Check sheet for the modelled part. Datum: model origin and axes. Units: mm. Give positions to 0.01 mm unless a question says otherwise; leave off trailing zeros. Loops run counter-clockwise (first coordinate to the right, second up) from the corner with the lowest first, then second, coordinate; pieces in that order, holes last. Notation, with made-up numbers: M 51.25,62 L 87.25,62 A19 ccw 87.25,82 Z; hole C 54,-14 d9. An arc over 180 degrees is marked long. Use one line per item in the form item = value.
from build123d import *

# Parameters (mm, degrees)
SKETCH1_R           = 75
BOSS_EXTRUDE1_DEPTH = 3.175
CUT_EXTRUDE1_DEPTH  = 3.175
SKETCH3_R           = 1.5875
CUT_EXTRUDE2_DEPTH  = 3.175
SKETCH4_R           = 27.051
CUT_EXTRUDE3_DEPTH  = 3.175
CUT_EXTRUDE4_DEPTH  = 3.175


with BuildPart() as part:
    # Sketch1 → Boss-Extrude1 (new body)
    with BuildSketch(Plane(origin=(0, 0, 0), x_dir=(1, 0, 0), z_dir=(0, 1, 0))):
        Circle(SKETCH1_R)
    extrude(amount=BOSS_EXTRUDE1_DEPTH)

    # Sketch2 → Cut-Extrude1 (cut)
    with BuildSketch(Plane(origin=(0, 3.175, 0), x_dir=(1, 0, 0), z_dir=(0, 1, 0))):
        with BuildLine():
            Line((-56.262005909, -49.594220339), (56.262005909, -49.594220339))
            ThreePointArc((56.262005909, -49.594220339), (0, -75), (-56.262005909, -49.594220339))
        make_face()
        with BuildLine():
            Line((-56.262005909, 49.594220339), (56.262005909, 49.594220339))
            ThreePointArc((56.262005909, 49.594220339), (0, 75), (-56.262005909, 49.594220339))
        make_face()
    extrude(amount=-CUT_EXTRUDE1_DEPTH, mode=Mode.SUBTRACT)

    # Sketch3 → Cut-Extrude2 (cut)
    with BuildSketch(Plane(origin=(0, 3.175, 0), x_dir=(1, 0, 0), z_dir=(0, 1, 0))):
        with Locations((-52.180304588, 44.729838125)):
            Circle(SKETCH3_R)
        with Locations((-19.05, 44.729838125)):
            Circle(SKETCH3_R)
        with Locations((19.05, 44.729838125)):
            Circle(SKETCH3_R)
        with Locations((52.180304588, 44.729838125)):
            Circle(SKETCH3_R)
        with Locations((52.180304588, -44.729838125)):
            Circle(SKETCH3_R)
        with Locations((19.05, -44.729838125)):
            Circle(SKETCH3_R)
        with Locations((-19.05, -44.729838125)):
            Circle(SKETCH3_R)
        with Locations((-52.180304588, -44.729838125)):
            Circle(SKETCH3_R)
    extrude(amount=-CUT_EXTRUDE2_DEPTH, mode=Mode.SUBTRACT)

    # Sketch4 → Cut-Extrude3 (cut)
    with BuildSketch(Plane(origin=(0, 3.175, 0), x_dir=(1, 0, 0), z_dir=(0, 1, 0))):
        with BuildLine():
            Line((-47.315937317, 44.741895283), (-23.177806764, 24.050282215))
            ThreePointArc((-23.177806764, 24.050282215), (-19.742091457, 26.942097653), (-15.949506316, 29.346891646))
            Line((-15.949506316, 29.346891646), (-20.527078848, 40.095137229))
            ThreePointArc((-20.527078848, 40.095137229), (-22.980849122, 41.864416778), (-23.914367271, 44.741895283))
            Line((-23.914367271, 44.741895283), (-47.315937317, 44.741895283))
        make_face()
        with BuildLine():
            ThreePointArc((10.107278818, 31.835039122), (0, 33.401), (-10.107278818, 31.835039122))
            Line((-10.107278818, 31.835039122), (-14.68485135, 42.583284705))
            ThreePointArc((-14.68485135, 42.583284705), (-14.312069768, 43.627916425), (-14.185617786, 44.729838125))
            Line((-14.185617786, 44.729838125), (14.185617786, 44.729838125))
            ThreePointArc((14.185617786, 44.729838125), (14.312069768, 43.627916425), (14.68485135, 42.583284705))
            Line((14.68485135, 42.583284705), (10.107278818, 31.835039122))
        make_face()
        with BuildLine():
            ThreePointArc((15.949506316, 29.346891646), (19.742091457, 26.942097653), (23.177806764, 24.050282215))
            Line((23.177806764, 24.050282215), (47.315937317, 44.741895283))
            Line((47.315937317, 44.741895283), (23.914382214, 44.729838125))
            ThreePointArc((23.914382214, 44.729838125), (22.977294896, 41.859547352), (20.527078848, 40.095137229))
            Line((20.527078848, 40.095137229), (15.949506316, 29.346891646))
        make_face()
        Circle(SKETCH4_R)
        with BuildLine():
            Line((-23.177806764, -24.050282215), (-47.315937317, -44.741895283))
            Line((-47.315937317, -44.741895283), (-23.914382214, -44.729838125))
            ThreePointArc((-23.914382214, -44.729838125), (-22.977294896, -41.859547352), (-20.527078848, -40.095137229))
            Line((-20.527078848, -40.095137229), (-15.949506316, -29.346891646))
            ThreePointArc((-15.949506316, -29.346891646), (-19.742091457, -26.942097653), (-23.177806764, -24.050282215))
        make_face()
        with BuildLine():
            ThreePointArc((-10.107278818, -31.835039122), (0, -33.401), (10.107278818, -31.835039122))
            Line((10.107278818, -31.835039122), (14.68485135, -42.583284705))
            ThreePointArc((14.68485135, -42.583284705), (14.312069768, -43.627916425), (14.185617786, -44.729838125))
            Line((14.185617786, -44.729838125), (-14.185617786, -44.729838125))
            ThreePointArc((-14.185617786, -44.729838125), (-14.312069768, -43.627916425), (-14.68485135, -42.583284705))
            Line((-14.68485135, -42.583284705), (-10.107278818, -31.835039122))
        make_face()
        with BuildLine():
            ThreePointArc((23.177806764, -24.050282215), (19.742091457, -26.942097653), (15.949506316, -29.346891646))
            Line((15.949506316, -29.346891646), (20.527078848, -40.095137229))
            ThreePointArc((20.527078848, -40.095137229), (22.977294896, -41.859547352), (23.914382214, -44.729838125))
            Line((23.914382214, -44.729838125), (47.315937317, -44.741895283))
            Line((47.315937317, -44.741895283), (23.177806764, -24.050282215))
        make_face()
    extrude(amount=-CUT_EXTRUDE3_DEPTH, mode=Mode.SUBTRACT)

    # Sketch5 → Cut-Extrude4 (cut)
    with BuildSketch(Plane(origin=(0, 3.175, 0), x_dir=(1, 0, 0), z_dir=(0, 1, 0))):
        with BuildLine():
            Line((58.957481542, 46.357473725), (27.31053772, 19.229179141))
            ThreePointArc((27.31053772, 19.229179141), (33.401, 0), (27.31053772, -19.229179141))
            Line((27.31053772, -19.229179141), (58.957481542, -46.357473725))
            ThreePointArc((58.957481542, -46.357473725), (75, 0), (58.957481542, 46.357473725))
        make_face()
        with BuildLine():
            Line((-54.190960711, 42.271531589), (-27.31053772, 19.229179141))
            ThreePointArc((-27.31053772, 19.229179141), (-33.401, 0), (-27.31053772, -19.229179141))
            Line((-27.31053772, -19.229179141), (-54.190960711, -42.271531589))
            ThreePointArc((-54.190960711, -42.271531589), (-68.728033622, 0), (-54.190960711, 42.271531589))
        make_face()
    extrude(amount=-CUT_EXTRUDE4_DEPTH, mode=Mode.SUBTRACT)


solid = part.part
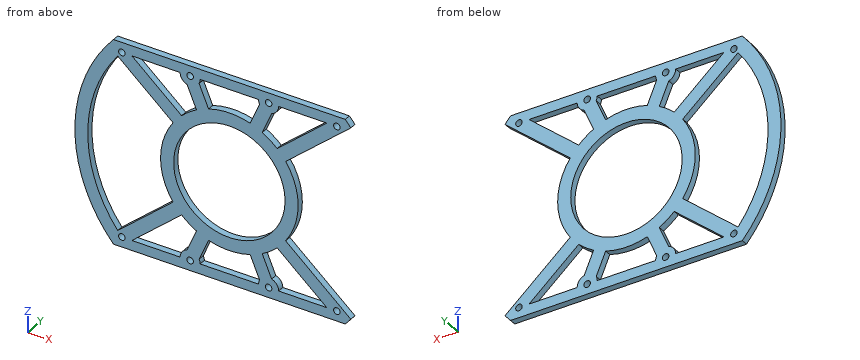
1) Scan lines: line 1 (Z direction, x = 0, y = 1.25); line 2 (Z direction, x = -23.5, y = 1.9); line 3 (X direction, y = 3, z = 8.5). Record each from-to range of solid material in increasing order.
Evaluation:
line_1 = -49.59 to -44.73, -33.4 to -27.05, 27.05 to 33.4, 44.73 to 49.59
line_2 = -49.59 to -42.77, -24.33 to -13.4, 13.4 to 24.33, 42.77 to 49.59
line_3 = -74.52 to -68.2, -32.3 to -25.68, 25.68 to 32.3
2) Section check B-B (z = -16). Record the cut outline in (x, y) (3 decimals), then the cut area to 3 significant figures.
Evaluation:
outline = M -73.273,0 L -66.84,0 L -66.84,3.175 L -73.273,3.175 Z; M -29.319,0 L -21.812,0 L -21.812,3.175 L -29.319,3.175 Z; M 21.812,0 L 29.319,0 L 29.319,3.175 L 21.812,3.175 Z
area = 68.1 mm^2
3) Depth check by flat-ended pin: pin 1 Ø2.5 at (x, z) = (-19.05, -44.73) entering from +Y; pin 2 Ø1 at (x, y) = (-61, 2.5) entering from +Z. Enter the tip coordinate at first touch or a pass-through.
Evaluation:
pin_1 = through
pin_2 = 44.33
4) Section check A-A (x = 0). Record the cut outline in (y, z) (3 decimals).
Evaluation:
outline = M 0,-49.594 L 3.175,-49.594 L 3.175,-44.73 L 0,-44.73 Z; M 0,-33.401 L 3.175,-33.401 L 3.175,-27.051 L 0,-27.051 Z; M 0,27.051 L 3.175,27.051 L 3.175,33.401 L 0,33.401 Z; M 0,44.73 L 3.175,44.73 L 3.175,49.594 L 0,49.594 Z
5) Section check D-D (x = 19.05). Record the cut outline in (y, z) (3 decimals).
Evaluation:
outline = M 0,-49.594 L 3.175,-49.594 L 3.175,-46.317 L 0,-46.317 Z; M 0,-43.142 L 3.175,-43.142 L 3.175,-36.627 L 0,-36.627 Z; M 0,-27.436 L 3.175,-27.436 L 3.175,-19.206 L 0,-19.206 Z; M 0,19.206 L 3.175,19.206 L 3.175,27.436 L 0,27.436 Z; M 0,36.627 L 3.175,36.627 L 3.175,43.142 L 0,43.142 Z; M 0,46.317 L 3.175,46.317 L 3.175,49.594 L 0,49.594 Z
6) Section check C-C (x = -29). Record the cut outline in (y, z) (3 decimals).
Evaluation:
outline = M 0,-49.594 L 3.175,-49.594 L 3.175,-44.742 L 0,-44.742 Z; M 0,-29.041 L 3.175,-29.041 L 3.175,-20.677 L 0,-20.677 Z; M 0,-16.572 L 3.175,-16.572 L 3.175,16.572 L 0,16.572 Z; M 0,20.677 L 3.175,20.677 L 3.175,29.041 L 0,29.041 Z; M 0,44.732 L 3.175,44.732 L 3.175,49.594 L 0,49.594 Z
